The model under review builds one solid part; all positions refer to its coordinate system, in mm. A direction names the side the tool comes from. Coordinates: 2 decimals unless noted, no trailing zeros. One line per item, written item: value.
```python
from build123d import *

# Parameters (mm, degrees)
BOSS_EXTRUDE1_DEPTH = 45
SKETCH2_R           = 11
CUT_EXTRUDE1_DEPTH  = 15
SKETCH4_R           = 200
CUT_EXTRUDE2_DEPTH  = 17.5
FILLET1_R           = 8
FILLET2_R           = 10
FILLET3_R           = 10


with BuildPart() as part:
    # Sketch1 → Boss-Extrude1 (new body)
    with BuildSketch(Plane(origin=(0, 0, 0), x_dir=(1, 0, 0), z_dir=(0, 1, 0))):
        with BuildLine():
            Line((-82, 13), (82, 13))
            ThreePointArc((82, 13), (95, 0), (82, -13))
            Line((82, -13), (-82, -13))
            ThreePointArc((-82, -13), (-95, 0), (-82, 13))
        make_face()
    extrude(amount=-BOSS_EXTRUDE1_DEPTH)

    # Sketch2 → Cut-Extrude1 (cut)
    with BuildSketch(Plane.XZ.offset(45)):
        with Locations(Location((-54, 0, 0), (0, 0, 270))):
            Circle(SKETCH2_R)
        with Locations(Location((54, 0, 0), (0, 0, 270))):
            Circle(SKETCH2_R)
    extrude(amount=-CUT_EXTRUDE1_DEPTH, mode=Mode.SUBTRACT)

    # Sketch4 → Cut-Extrude2 (cut, symmetric)
    with BuildSketch(Plane.XY):
        with Locations((0.724830201, 185)):
            Circle(SKETCH4_R)
    extrude(amount=CUT_EXTRUDE2_DEPTH, both=True, mode=Mode.SUBTRACT)

    # Fillet1
    # the kernel refuses this fillet: 8 mm, written as the material it takes off along each edge
    with BuildSketch(Plane(origin=(82, -45, 0), x_dir=(0, 0, -1), z_dir=(-1, 0, 0))) as fillet1_piece_1:
        with BuildLine():
            CenterArc((13 - FILLET1_R, -FILLET1_R), FILLET1_R, 0, 90)
            Line((13, -FILLET1_R), (13, 0))
            Line((13, 0), (13 - FILLET1_R, 0))
        make_face()
    revolve(axis=Axis((82, -45, 0), (0, -1, 0)), revolution_arc=180, mode=Mode.SUBTRACT)
    with BuildSketch(Plane(origin=(-82, -45, -13), x_dir=(0, 0, 1), z_dir=(1, 0, 0))) as fillet1_piece_2:
        with BuildLine():
            CenterArc((FILLET1_R, -FILLET1_R), FILLET1_R, 90, 90)
            Line((0, -FILLET1_R), (0, 0))
            Line((0, 0), (FILLET1_R, 0))
        make_face()
    extrude(amount=164, mode=Mode.SUBTRACT)
    with BuildSketch(Plane(origin=(-82, -45, 0), x_dir=(0, 0, 1), z_dir=(1, 0, 0))) as fillet1_piece_3:
        with BuildLine():
            CenterArc((13 - FILLET1_R, -FILLET1_R), FILLET1_R, 0, 90)
            Line((13 - FILLET1_R, 0), (13, 0))
            Line((13, 0), (13, -FILLET1_R))
        make_face()
    revolve(axis=Axis((-82, -45, 0), (0, -1, 0)), revolution_arc=180, mode=Mode.SUBTRACT)
    with BuildSketch(Plane(origin=(82, -45, 13), x_dir=(0, 1, 0), z_dir=(-1, 0, 0))) as fillet1_piece_4:
        with BuildLine():
            CenterArc((FILLET1_R, FILLET1_R), FILLET1_R, 180, 90)
            Line((0, FILLET1_R), (0, 0))
            Line((0, 0), (FILLET1_R, 0))
        make_face()
    extrude(amount=164, mode=Mode.SUBTRACT)

    # Fillet2
    # the kernel refuses this fillet: 10 mm, written as the material it takes off along each edge
    with BuildSketch(Plane(origin=(82, 0, 13), x_dir=(0, -1, 0), z_dir=(-1, 0, 0))) as fillet2_piece_1:
        with BuildLine():
            CenterArc((FILLET2_R, -FILLET2_R), FILLET2_R, 90, 90)
            Line((0, -FILLET2_R), (0, 0))
            Line((0, 0), (FILLET2_R, 0))
        make_face()
    extrude(amount=30.281749031, mode=Mode.SUBTRACT)
    with BuildSketch(Plane(origin=(-82, 0, -13), x_dir=(0, 0, 1), z_dir=(1, 0, 0))) as fillet2_piece_2:
        with BuildLine():
            CenterArc((FILLET2_R, FILLET2_R), FILLET2_R, 180, 90)
            Line((0, FILLET2_R), (0, 0))
            Line((0, 0), (FILLET2_R, 0))
        make_face()
    extrude(amount=31.731409434, mode=Mode.SUBTRACT)
    with BuildSketch(Plane(origin=(0.724830201, 185, -13), x_dir=(-0.49233736380683973, -0.8704044578239082, 0), z_dir=(-0.8704044578239082, 0.49233736380683973, 0))) as fillet2_piece_3:
        with BuildLine():
            CenterArc((200 + FILLET2_R, FILLET2_R), FILLET2_R, 180, 90)
            Line((200 + FILLET2_R, 0), (200, 0))
            Line((200, 0), (200, FILLET2_R))
        make_face()
    revolve(axis=Axis((0.724830201, 185, -13), (0, 0, 1)), revolution_arc=58.988651661, mode=Mode.SUBTRACT)
    with BuildSketch(Plane(origin=(0.724830201, 185, 13), x_dir=(-0.49233736380683973, -0.8704044578239082, 0), z_dir=(-0.8704044578239082, 0.49233736380683973, 0))) as fillet2_piece_4:
        with BuildLine():
            CenterArc((200 + FILLET2_R, -FILLET2_R), FILLET2_R, 90, 90)
            Line((200, -FILLET2_R), (200, 0))
            Line((200, 0), (200 + FILLET2_R, 0))
        make_face()
    revolve(axis=Axis((0.724830201, 185, 13), (0, 0, 1)), revolution_arc=58.988651661, mode=Mode.SUBTRACT)
    with BuildSketch(Plane(origin=(51.718250969, 0, -13), x_dir=(0, 0, 1), z_dir=(1, 0, 0))) as fillet2_piece_5:
        with BuildLine():
            CenterArc((FILLET2_R, FILLET2_R), FILLET2_R, 180, 90)
            Line((0, FILLET2_R), (0, 0))
            Line((0, 0), (FILLET2_R, 0))
        make_face()
    extrude(amount=30.281749031, mode=Mode.SUBTRACT)
    with BuildSketch(Plane(origin=(82, 0, 0), x_dir=(0, 0, -1), z_dir=(-1, 0, 0))) as fillet2_piece_6:
        with BuildLine():
            CenterArc((13 - FILLET2_R, FILLET2_R), FILLET2_R, 270, 90)
            Line((13, FILLET2_R), (13, 0))
            Line((13, 0), (13 - FILLET2_R, 0))
        make_face()
    revolve(axis=Axis((82, 0, 0), (0, -1, 0)), revolution_arc=180, mode=Mode.SUBTRACT)
    with BuildSketch(Plane(origin=(-50.268590566, 0, 13), x_dir=(0, -1, 0), z_dir=(-1, 0, 0))) as fillet2_piece_7:
        with BuildLine():
            CenterArc((FILLET2_R, -FILLET2_R), FILLET2_R, 90, 90)
            Line((0, -FILLET2_R), (0, 0))
            Line((0, 0), (FILLET2_R, 0))
        make_face()
    extrude(amount=31.731409434, mode=Mode.SUBTRACT)
    with BuildSketch(Plane(origin=(-82, 0, 0), x_dir=(0, 0, 1), z_dir=(1, 0, 0))) as fillet2_piece_8:
        with BuildLine():
            CenterArc((13 - FILLET2_R, FILLET2_R), FILLET2_R, 270, 90)
            Line((13, FILLET2_R), (13, 0))
            Line((13, 0), (13 - FILLET2_R, 0))
        make_face()
    revolve(axis=Axis((-82, 0, 0), (0, -1, 0)), revolution_arc=180, mode=Mode.SUBTRACT)

    # Fillet3
    fillet3_edges = [part.edges().sort_by_distance(p)[0] for p in [
        (-75.268590566, 0, 0),
        (76.718250969, 0, 0),
        (77.300565536, -2.961441402, 10.103428202),
        (-75.850905134, -2.961441403, 10.103428203),
        (77.300565536, -2.961441402, -10.103428202),
        (-75.850905134, -2.961441403, -10.103428203),
    ]]
    fillet(fillet3_edges, radius=FILLET3_R)


solid = part.part
```
(1) Mouldability with a two-part tool opening along X and no side actions: class faces 3 (the cylindrical face through (-50.696, -37.605, -10.492)), 4 (the cylindrical face through (-75.354, -0.175, 0.042)), 5 (the flat face through (1, -29, 13)), 6 (the cylindrical face through (95, -23, 0)) as +X half, -X half, draft (parallel to the pull), parting line (faces both ways), or undercut.
Geometry results:
face 3: undercut
face 4: undercut
face 5: draft
face 6: +X half
(2) For L1, parallel to X at y = -34, z = -0.25; L2, parallel to X at y = -40.5, z = 0; L3, parallel to Z at x = 54, y = -37, list the stretches that pass through material, from the lowest coordinate up.
Geometry results:
L1: x = -95 to -65, -43 to 43, 65 to 95
L2: x = -94.19 to -65, -43 to 43, 65 to 94.19
L3: z = -13 to -11, 11 to 13
(3) Insertion check: pin 1 Ø3 at (x, z) = (70, 8) entering from -Y; pin 2 Ø1.5 at (y, z) = (-30, 8.5) entering from +X; pin 3 Ø6 at (y, z) = (-14.5, -8) entering from +X. Each pin has a flat end and moves straight along its axis. Give the tip position at first contact, or say it passes through.
Geometry results:
pin 1: stops at y = -44.86
pin 2: stops at x = 92.44
pin 3: stops at x = 94
(4) Tool access review of faces 1 (the cylindrical face through (57.304, -37.605, -10.492)), 2 (the cylindrical face through (-1.148, -42.719, -10.594)): name each direction out of +Z, -Z, +X, -X, +Y, -Y from which nothing blocks a thin tool from reaching the whole face with its end or side.
Geometry results:
face 1: -Y
face 2: -Z, +X, -X, -Y
